Verification items for the finished model (mm, model axes). A direction names the side the tool comes from. Give positions to 0.01 mm unless a question says otherwise; leave off trailing zeros. Write each loop counter-clockwise with the first axis right and the second up, starting at its lowest first coordinate (ties: lowest second). Pieces come first, ordered by that corner, then holes. Notation, with made-up numbers: (89, 21) -> (148, 21) arc R32 cw to (148, 48) -> close; hole circle Ø1 at (29.5, 10). An arc over 180 degrees is marked (long way). Use one line per item in the form item = value. Start each with the question number.
(1) Section check B-B, the plane z = 0. State how many separate pieces and enclosed holes the cut face has, plus the area to 3 significant figures.
(2) Release check for a two-part mould opening along Y. For faces 3 (the face through (0, -4, -3)), 4 (the face through (46.999, -11.012, 14.362)), 5 (the face through (47.124, 15.046, -9.593)) record: pulls with the +Y half, pulls with the -Y half, needs draft (parallel to the pull), parting line crosses it, or undercut.
(3) Section check C-C, the plane x = 23. Record the cut outline in (y, z), plus the area to 3 significant figures.
(4) Depth check by flat-ended pin: pin 1 Ø0.9 at (y, z) = (-17, -1) entering from -X; pin 2 Ø1 at (x, y) = (28, -7.5) entering from -Z; pin 3 Ø12 at (x, z) = (38.5, -2.5) entering from -Y; pin 4 Ø6 at (x, y) = (40, -4) entering from -Z. Enter the tip coordinate at first touch or a pass-through.
(5) Scan lines: L1, parallel to Y at x = 20, z = 0; L2, parallel to Y at x = 47.2, z = 0. Record each from-to range of solid material in increasing order.
(6) Set-up check for faces 1 (the face through (46.609, -13, -12)), 2 (the face through (23.497, -17.763, -0.782)): record each of +Z, -Z, +X, -X, +Y, -Y from which the full face is reachable in a straight line by a thin tool's end or side.
Autodesk Inventor part; units mm, degrees
ref_plane "YZ Plane" through (0, 0, 0) normal (1, 0, 0) x (0, 1, 0)
ref_plane "XZ Plane" through (0, 0, 0) normal (0, 1, 0) x (-1, 0, 0)
ref_plane "XY Plane" through (0, 0, 0) normal (0, 0, 1) x (1, 0, 0)
sketch "Sketch1" plane through (0, 0, 0) normal (1, 0, 0) x (0, 1, 0)
  circle A0 centre (0, 0) radius 17.78
  dimension "d0" = 35.56
extrude "Extrusion1" add sketch "Sketch1" along normal blind 47.625
fillet "Fillet1" radius 1.27 1 edges at (0, -17.78, 0)
sketch "Sketch2" plane through (0, 0, 0) normal (0, 1, 0) x (-1, 0, 0)
  line L0 (-34.29, -7.9375) -> (-39.37, -7.9375)
  line L1 (-40.005, -7.3025) -> (-40.005, 7.3025)
  line L2 (-39.37, 7.9375) -> (-34.29, 7.9375)
  line L3 (-33.655, 7.3025) -> (-33.655, -7.3025)
  line L4 (-47.625, 17.78) -> (-47.625, -17.78)
  arc A0 (-40.005, -7.3025) -> (-39.37, -7.9375) centre (-39.37, -7.3025) ccw
  arc A1 (-34.29, -7.9375) -> (-33.655, -7.3025) centre (-34.29, -7.3025) ccw
  arc A2 (-33.655, 7.3025) -> (-34.29, 7.9375) centre (-34.29, 7.3025) ccw
  arc A3 (-39.37, 7.9375) -> (-40.005, 7.3025) centre (-39.37, 7.3025) ccw
  point P0 (0, 0)
  point P1 (-33.655, -7.9375)
  point P2 (-40.005, 7.9375)
  point P3 (-40.005, -7.9375)
  point P4 (-33.655, 7.9375)
  dimension "d4" = 15.875
  dimension "d5" = 6.35
  dimension "d6" = 7.62
  dimension "d7" = 9.8425
  dimension "d14" = 0.635
sketch "Sketch3" plane through (47.625, 0, 0) normal (1, 0, 0) x (0, 0, -1)
  circle A0 centre (0, 0) radius 18.0975
  dimension "d11" = 36.195
extrude "Extrusion3" add sketch "Sketch3" against normal blind 1.27
shell "Shell2" thickness 0.254 removed faces 1 at (47.625, -0.1965, 3.481)
extrude "Extrusion2" cut sketch "Sketch2" along normal up to next
sketch "Sketch4" plane through (0, 0, 0) normal (-1, 0, 0) x (0, 0, 1)
  circle A0 centre (0, 0) radius 4.7625
  dimension "d16" = 9.525
extrude "Extrusion4" cut sketch "Sketch4" against normal up to next
extrude "Extrusion5" cut sketch "Sketch2" against normal up to next
properties part number "Motor-Casing"
Completed:
q1.separate_pieces = 4
q1.enclosed_holes = 0
q1.area = 27.4 mm²
q2.face_3 = needs draft
q2.face_4 = parting line crosses it
q2.face_5 = undercut
q3.outline = circle Ø35.56 at (0, 0); hole circle Ø35.05 at (0, 0)
q3.area = 28.2 mm²
q4.pin_1 = 0
q4.pin_2 = -16.34
q4.pin_3 = -17.78
q4.pin_4 = -17.75
q5.L1 = -17.78 to -17.53, 17.53 to 17.78
q5.L2 = -18.1 to -17.84, 17.84 to 18.1
q6.face_1 = +X
q6.face_2 = -X
